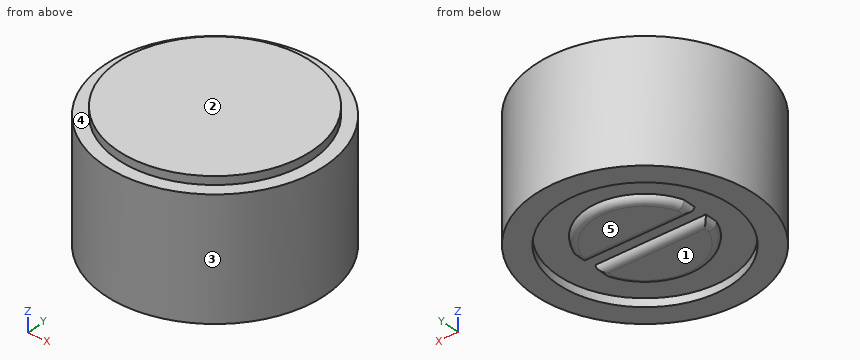
Autodesk Inventor part; units mm, degrees
ref_plane "YZ Plane" through (0, 0, 0) normal (1, 0, 0) x (0, 1, 0)
ref_plane "XZ Plane" through (0, 0, 0) normal (0, 1, 0) x (-1, 0, 0)
ref_plane "XY Plane" through (0, 0, 0) normal (0, 0, 1) x (1, 0, 0)
sketch "Sketch1" plane through (0, 0, 0) normal (0, 0, 1) x (1, 0, 0)
  circle A0 centre (0, 0) radius 4
  dimension "d0" = 8
extrude "Extrusion1" add sketch "Sketch1" along normal blind 4.35
sketch "Sketch2" plane through (0, 0, 4.35) normal (0, 0, 1) x (1, 0, 0)
  circle A0 centre (0, 0) radius 3.525
  circle A1 centre (0, 0) radius 4
  dimension "d16" = 7.05
extrude "Extrusion2" add sketch "Sketch2" along normal blind 0.3 contours A0
sketch "Sketch3" plane through (0, 0, 0) normal (0, 0, -1) x (-1, 0, 0)
  circle A0 centre (0, 0) radius 3.15
  circle A1 centre (0, 0) radius 4
  dimension "d17" = 6.3
extrude "Extrusion3" cut sketch "Sketch3" against normal blind 0.3 contours A0
sketch "Sketch4" plane through (0, 0, 0.3) normal (0, 0, -1) x (-1, 0, 0)
  arc A0 (2, 0.7181) -> (-2, 0.7181) centre (0, 0) ccw
  line L0 (2, 0.7181) -> (2, 0.25)
  line L1 (2, 0.25) -> (0, 0.25)
  line L2 (-2, 0.25) -> (-2, 0.7181)
  circle A1 centre (0, 0) radius 3.525 construction
  circle A2 centre (0, 0) radius 3.15 construction
  line L3 (0, 0) -> (0, 3.15) construction
  line L4 (0, 0.25) -> (-2, 0.25)
  line L5 (0, 0) -> (3.15, 0) construction
  arc A3 (-2, -0.7181) -> (2, -0.7181) centre (0, 0) ccw
  line L6 (2, -0.7181) -> (2, -0.25)
  line L7 (2, -0.25) -> (0, -0.25)
  line L8 (-2, -0.25) -> (-2, -0.7181)
  line L9 (0, -0.25) -> (-2, -0.25)
  dimension "d9" = 1.4
  dimension "d10" = 2
  dimension "d12" = 0.5
extrude "Extrusion4" add sketch "Sketch4" along normal blind 0.25
fillet "Fillet1" radius 0.25 8 edges at (0, 2.125, 0.05) (2, 0.484, 0.05) (0, 0.25, 0.05) (-2, 0.484, 0.05) (0, -0.25, 0.05) (2, -0.484, 0.05) (0, -2.125, 0.05) (-2, -0.484, 0.05)
equation "\"d9\" = leadInset"
equation "\"d10\" = 0.5 * leadWidth"
equation "\"d12\" = leadSeparation"
equation "\"d13\" = leadExtrusion"
equation "\"d15\" = leadExtrusion"
equation "\"membraneInset\" = 0.25"
equation "\"backplateInset\" = membraneInset"
equation "\"backplateExtrusion\" = 0.125"
equation "\"leadInset\" = 1.4"
equation "\"leadSeparation\" = 0.5"
equation "\"leadWidth\" = 4"
equation "\"leadExtrusion\" = 2 * backplateExtrusion"
properties part number "Mic_Unidirectional"
For this review, take the finished solid that the model builds, in its own axes (mm). Face numbers are marked on the shaded views. A direction names the side the tool comes from. Round coordinates to 2 decimals unless told otherwise and drop trailing zeros. Write each loop counter-clockwise with the first axis right and the second up, starting at its lowest first coordinate (ties: lowest second). Pieces come first, ordered by that corner, then holes. Notation, with made-up numbers: (80.5, 88.5) -> (85.5, 88.5) arc R15 ccw to (85.5, 111.5) -> close; hole circle Ø4 at (-12, 55). An arc over 180 degrees is marked (long way). Use one line per item in the form item = value.
Q1. To check wall thickness, follow probe 1 along Z at (x, y) = (1.5, 3.5); probe 2 along Z at (x, y) = (-2.75, 0); probe 3 along X at (y, z) = (2.25, 1.7). State the ranges of each line that lie inside material, in increasing order. Write a range as from..to.
Resolved:
probe_1 = 0..4.35
probe_2 = 0.3..4.65
probe_3 = -3.31..3.31
Q2. Consider section C-C (z = 2.1). State the section outline as (x, y) points.
Resolved:
outline = circle Ø8 at (0, 0)
Q3. Consider section A-A (y = 0). State the section outline as (x, z) points (3 decimals), then the cut area to 3 significant figures.
Resolved:
outline = (-4, 0) -> (-3.15, 0) -> (-3.15, 0.3) -> (3.15, 0.3) -> (3.15, 0) -> (4, 0) -> (4, 4.35) -> (3.525, 4.35) -> (3.525, 4.65) -> (-3.525, 4.65) -> (-3.525, 4.35) -> (-4, 4.35) -> close
area = 35.0 mm²
Q4. Clearance check with flat-ended pins moving along their axes: pin 1 Ø2 at (x, z) = (3, 2.5) entering from +Y; pin 2 Ø0.7 at (x, y) = (0, -1.5) entering from -Z; pin 3 Ø1 at (y, z) = (-1, 3.5) entering from -X. State where each tip first meets the part, or that it passes through.
Resolved:
pin_1 = 3.46
pin_2 = 0.05
pin_3 = -3.97
Q5. Consider section D-D (y = 2.25). State the section outline as (x, z) points.
Resolved:
outline = (-3.31, 0) -> (-2.2, 0) -> (-2.2, 0.3) -> (2.2, 0.3) -> (2.2, 0) -> (3.31, 0) -> (3.31, 4.35) -> (2.71, 4.35) -> (2.71, 4.65) -> (-2.71, 4.65) -> (-2.71, 4.35) -> (-3.31, 4.35) -> close
Q6. The part is to be moulded in two halves that separate along X. For the marked faces 3, 4 and 5, say which applies: released by +X, released by -X, zero draft, split by the parting line, or undercut.
Resolved:
face_3 = split by the parting line
face_4 = zero draft
face_5 = undercut
Q7. Machinability: for the marked faces 1 and 2, which of the approach directions +Z, -Z, +X, -X, +Y, -Y give a long, thin tool a straight path to every point of the face, cutting with its end or side? Answer none if there is none.
Resolved:
face_1 = -Z
face_2 = +Z, +X, -X, +Y, -Y
